Autodesk Inventor part; units mm, degrees
ref_plane "YZ Plane" through (0, 0, 0) normal (1, 0, 0) x (0, 1, 0)
ref_plane "XZ Plane" through (0, 0, 0) normal (0, 1, 0) x (-1, 0, 0)
ref_plane "XY Plane" through (0, 0, 0) normal (0, 0, 1) x (1, 0, 0)
sketch "スケッチ1" plane through (0, 0, 0) normal (1, 0, 0) x (0, 1, 0)
  line L0 (-65, 20) -> (65, 20)
  line L1 (65, 20) -> (65, -20)
  line L2 (65, -20) -> (-65, -20)
  line L3 (-65, -20) -> (-65, 20)
  line L4 (-65, 20) -> (65, -20) construction
  line L5 (65, 20) -> (-65, -20) construction
  line L6 (65, -20) -> (65, -70)
  line L7 (65, -70) -> (15, -70)
  line L8 (15, -70) -> (0, -45)
  line L9 (-10, -45) -> (-25, -70)
  line L10 (-25, -70) -> (-65, -70)
  line L11 (-65, -70) -> (-65, -20)
  line L12 (0, -45) -> (-10, -45)
  line L13 (0, -20) -> (-10, -20)
  line L14 (-10, -20) -> (-10, -45)
  line L15 (-10, -45) -> (0, -45)
  line L16 (0, -45) -> (0, -20)
  point P0 (0, 0)
  point P1 (-5, -45)
  point P2 (0, 0)
  point P3 (0, -45)
  dimension "d0" = 130
  dimension "d1" = 40
  dimension "d18" = 50
  dimension "d19" = 50
  dimension "d22" = 5
  dimension "d24" = 25
  dimension "d25" = 10
extrude "押し出し1" add sketch "スケッチ1" along normal blind 5 contours L0 L1 L2 L3 | L2 L14 L9 L10 L11 | L6 L7 L8 L16 L2
sketch "スケッチ3" plane through (5, 0, 0) normal (1, 0, 0) x (0, 0, -1)
  line L0 (-10, 3.5) -> (5, 3.5)
  line L1 (5, 3.5) -> (5, 4.5)
  line L2 (5, 4.5) -> (-10, 4.5)
  line L3 (-10, 4.5) -> (-10, 3.5)
  line L4 (-15, 0) -> (10, 0)
  line L5 (10, 0) -> (10, 8)
  line L6 (10, 8) -> (-15, 8)
  line L7 (-15, 8) -> (-15, 0)
  line L8 (-20, 65) -> (-20, -65)
  point P0 (0, 0)
  point P1 (-2.5, 8)
  point P2 (-2.5, 4.5)
  point P3 (-10, 4)
  point P4 (-15, 4)
  dimension "d7" = 15
  dimension "d8" = 1
  dimension "d9" = 25
  dimension "d10" = 8
  dimension "d17" = 5
extrude "押し出し3" cut sketch "スケッチ3" against normal through all contours L3 L2 L1 L0
chamfer "面取り1" distance 5 angle 45 1 edges at (5, 0, 20)
properties part number "VertMove" material "スタイロフォームIB"
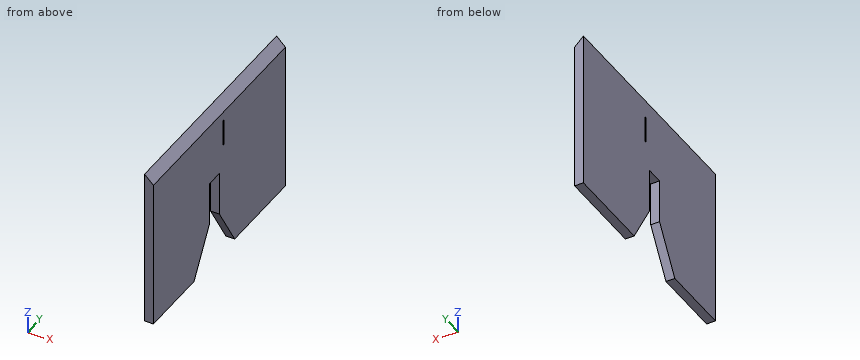
Geometry: final body of the model. Coordinates: model frame, mm. Coordinates: 2 decimals unless noted, no trailing zeros. Loops run counter-clockwise (first coordinate to the right, second up) from the corner with the lowest first, then second, coordinate; pieces in that order, holes last. Notation, with made-up numbers: M 53,58.25 L 102,58.25 A36 ccw 102,97.25 Z; hole C 73.25,-26.5 d10. An arc over 180 degrees is marked long. One line per item, written item: value. Start each with the question number.
1) Cut plane D-D (z = -53). Return loops of the section in (x, y).
2) Material intervals for L1, parallel to Y at x = 1.3, z = 7; L2, parallel to Y at x = 1.1, z = -45; L3, parallel to Z at x = 3.05, y = -40, sorted ascending. Write a range as from..to.
3) Pin query (flat end, axial travel): P1, Ø1.1, axis at x = 2.5, y = 4, coming from the +Z side. Return the tip coordinate at first contact, or that it passes through.
4) Cut plane B-B (x = 2.6). Return loops of the section in (y, z).
5) Cut plane A-A (z = -28). Return loops of the section in (x, y), then the cut area to 3 significant figures.
Evaluation:
1. outline: M 0,-65 L 5,-65 L 5,-14.8 L 0,-14.8 Z; M 0,4.8 L 5,4.8 L 5,65 L 0,65 Z
2. L1: -65..3.5, 4.5..65
2. L2: -65..-10, 0..65
2. L3: -70..16.95
3. P1: z = 18.05
4. outline: M -65,-70 L -25,-70 L -10,-45 L -10,-20 L 0,-20 L 0,-45 L 15,-70 L 65,-70 L 65,17.4 L -65,17.4 Z; hole M 3.5,-5 L 4.5,-5 L 4.5,10 L 3.5,10 Z
5. outline: M 0,-65 L 5,-65 L 5,-10 L 0,-10 Z; M 0,0 L 5,0 L 5,65 L 0,65 Z
5. area: 600 mm^2
